from build123d import *

# Parameters (mm, degrees)
BOSS_EXTRUDE1_DEPTH         = 12.7
BOSS_EXTRUDE1_DEPTH_BACK    = 12.7
SKETCH2_W                   = 34.908195051
SKETCH2_H                   = 15.24
CUT_EXTRUDE1_DEPTH          = 38.1
F_1_4_CLEARANCE_HOLE1_D     = 6.7564
F_1_4_CLEARANCE_HOLE1_DEPTH = 25.4
F_1_4_CLEARANCE_HOLE1_TIP   = 2.029827343


with BuildPart() as part:
    # Sketch1 → Boss-Extrude1 (new body, two sides)
    with BuildSketch(Plane.XY) as boss_extrude1_sk:
        Polygon((556.99412228, -1558.656635977), (556.99412228, -1577.490689714), (588.727317331, -1587.123662845), (601.427317331, -1587.123662845), (601.427317331, -1549.023662845), (588.727317331, -1549.023662845), align=None)
    extrude(amount=BOSS_EXTRUDE1_DEPTH)
    extrude(boss_extrude1_sk.sketch, amount=-BOSS_EXTRUDE1_DEPTH_BACK)

    # Sketch2 → Cut-Extrude1 (cut)
    with BuildSketch(Plane.XZ.offset(1587.123662845)):
        with Locations((574.448219806, 0)):
            Rectangle(SKETCH2_W, SKETCH2_H)
    extrude(amount=-CUT_EXTRUDE1_DEPTH, mode=Mode.SUBTRACT)

    # 1/4 Clearance Hole1
    with Locations(Plane.XY.offset(12.7)):
        with Locations((569.69412228, -1568.073662845)):
            Hole(F_1_4_CLEARANCE_HOLE1_D / 2, depth=F_1_4_CLEARANCE_HOLE1_DEPTH)
            with Locations((0, 0, -(F_1_4_CLEARANCE_HOLE1_DEPTH + F_1_4_CLEARANCE_HOLE1_TIP / 2))):  # 118° drill point
                Cone(0, F_1_4_CLEARANCE_HOLE1_D / 2, F_1_4_CLEARANCE_HOLE1_TIP, mode=Mode.SUBTRACT)


solid = part.part
The listing builds one solid part. Answer for the finished solid, in the listing's coordinates (mm). A direction names the side the tool comes from. Give positions to 0.01 mm unless a question says otherwise; leave off trailing zeros. Write each loop counter-clockwise with the first axis right and the second up, starting at its lowest first coordinate (ties: lowest second). Pieces come first, ordered by that corner, then holes. Notation, with made-up numbers: (-36.75, 6) -> (-4.75, 6) arc R23 cw to (-4.75, 41) -> close; hole circle Ø3 at (66, 66). An arc over 180 degrees is marked (long way). Use a Markdown table: item, result.
(1) Find the intervals of material crossed by probe 1 along Z at (x, y) = (590.5, -1568.5); probe 2 along Y at (x, z) = (569.5, 10.5); probe 3 along X at (y, z) = (-1572, 7.25), in increasing order. Write a range as from..to.
Return value:
| item | result |
|---|---|
| probe 1 | -12.7..-7.62, 7.62..12.7 |
| probe 2 | -1581.29..-1571.45, -1564.7..-1554.86 |
| probe 3 | 591.9..601.43 |
(2) Determine the mould class of faces 3 (the flat face through (573.083, -1553.773, 10.196)), 4 (the flat face through (578, -1568, -7.62)), 5 (the cylindrical face through (568.135, -1571.071, -10.196)) for opening direction Y: released by +Y, released by -Y, zero draft, split by the parting line, or undercut.
Return value:
| item | result |
|---|---|
| face 3 | released by +Y |
| face 4 | zero draft |
| face 5 | undercut |
(3) Section A-A, the plane y = -1565.5 is taken. Determine the outline of the cut face in (x, z).
Return value:
| item | result |
|---|---|
| outline | (556.99, -12.7) -> (567.51, -12.7) -> (567.51, -7.62) -> (556.99, -7.62) -> close; (556.99, 7.62) -> (567.51, 7.62) -> (567.51, 12.7) -> (556.99, 12.7) -> close; (571.88, -12.7) -> (601.43, -12.7) -> (601.43, 12.7) -> (571.88, 12.7) -> (571.88, 7.62) -> (591.9, 7.62) -> (591.9, -7.62) -> (571.88, -7.62) -> close |
(4) Section C-C, the plane y = -1572.5 is taken. Determine the outline of the cut face in (x, z), then the cut area to 3 significant figures.
Return value:
| item | result |
|---|---|
| outline | (556.99, -12.7) -> (601.43, -12.7) -> (601.43, 12.7) -> (556.99, 12.7) -> (556.99, 7.62) -> (591.9, 7.62) -> (591.9, -7.62) -> (556.99, -7.62) -> close |
| area | 597 mm2 |
(5) Section D-D, the plane x = 581.5 is taken. Determine the outline of the cut face in (y, z).
Return value:
| item | result |
|---|---|
| outline | (-1584.93, -12.7) -> (-1551.22, -12.7) -> (-1551.22, -7.62) -> (-1584.93, -7.62) -> close; (-1584.93, 7.62) -> (-1551.22, 7.62) -> (-1551.22, 12.7) -> (-1584.93, 12.7) -> close |
(6) For faces 1 (the flat face through (591.902, -1568, 0)), 2 (the flat face through (572.64, -1582.24, 10.2)), determine the directions among +Z, -Z, +X, -X, +Y, -Y from which every point of the face is accessible in a straight line to the end or side of a thin tool.
Return value:
| item | result |
|---|---|
| face 1 | -X, +Y, -Y |
| face 2 | +Z, -Z, -X, -Y |
(7) Flat-ended cylindrical pins translate along their axes: P1, Ø6, axis at x = 574, z = 7.5, coming from the -Y side; P2, Ø8, axis at y = -1554, z = -0.5, coming from the -X side; P3, Ø1.5, axis at x = 572.5, z = 7.5, coming from the +Y side. Find the tip coordinate at first contact, or state that the pin passes through.
Return value:
| item | result |
|---|---|
| P1 | y = -1583.56 |
| P2 | x = 591.9 |
| P3 | y = -1553.72 |
(8) Section B-B, the plane x = 568 is taken. Determine the outline of the cut face in (y, z).
Return value:
| item | result |
|---|---|
| outline | (-1580.83, -12.7) -> (-1571, -12.7) -> (-1571, -7.62) -> (-1580.83, -7.62) -> close; (-1580.83, 7.62) -> (-1571, 7.62) -> (-1571, 12.7) -> (-1580.83, 12.7) -> close; (-1565.15, -12.7) -> (-1555.32, -12.7) -> (-1555.32, -7.62) -> (-1565.15, -7.62) -> close; (-1565.15, 7.62) -> (-1555.32, 7.62) -> (-1555.32, 12.7) -> (-1565.15, 12.7) -> close |
